Geometry: final body of the model. Coordinates: model frame, mm. Face numbers are marked on the shaded views. A direction names the side the tool comes from. Give positions to 0.01 mm unless a question says otherwise; leave off trailing zeros. Loops run counter-clockwise (first coordinate to the right, second up) from the corner with the lowest first, then second, coordinate; pieces in that order, holes last.
from build123d import *

# Parameters (mm, degrees)
F1_DEPTH = 25.4
F2_R     = 3.425
F3_DEPTH = 25.4
F4_R     = 5.08
F6_DEPTH = 6.35


with BuildPart() as f1:
    # F0 (on Top) → F1 (new body)
    with BuildSketch(Plane.XY):
        with BuildLine():
            ThreePointArc((-17.6783595035, -30.6198168546), (0, -27.3250688074), (17.6783595035, -30.6198168546))
            ThreePointArc((17.6783595035, -30.6198168546), (23.6642037473, -13.6625344037), (35.3567190071, 0))
            ThreePointArc((35.3567190071, 0), (23.6642037473, 13.6625344037), (17.6783595035, 30.6198168546))
            ThreePointArc((17.6783595035, 30.6198168546), (0, 27.3250688074), (-17.6783595035, 30.6198168546))
            ThreePointArc((-17.6783595035, 30.6198168546), (-23.6642037473, 13.6625344037), (-35.3567190071, 0))
            ThreePointArc((-35.3567190071, 0), (-23.6642037473, -13.6625344037), (-17.6783595035, -30.6198168546))
        make_face()
    extrude(amount=F1_DEPTH)

    # F2 (on face) → F3 (cut)
    with BuildSketch(Plane.XY.offset(25.4)):
        Circle(F2_R)
    extrude(amount=-F3_DEPTH, mode=Mode.SUBTRACT)

    # F4
    f4_edges = [f1.edges().sort_by_distance(p)[0] for p in [
        (-35.356719, 0, 12.7),
        (-17.67836, -30.619817, 12.7),
        (17.67836, -30.619817, 12.7),
        (35.356719, 0, 12.7),
        (17.67836, 30.619817, 12.7),
        (-17.67836, 30.619817, 12.7),
        (0, -27.325069, 0),
        (-23.664204, -13.662534, 0),
        (23.664204, -13.662534, 0),
        (-23.664204, 13.662534, 0),
        (23.664204, 13.662534, 0),
        (0, 27.325069, 0),
        (-3.425, 0, 0),
    ]]
    fillet(f4_edges, radius=F4_R)

    # F5 (on face) → F6 (cut)
    with BuildSketch(Plane.XY.offset(25.4)):
        Polygon((-1.9887100499, -6.5160084155), (4.6486737941, -4.9802776317), (6.637383844, 1.5357307838), (1.9887100499, 6.5160084155), (-4.6486737941, 4.9802776317), (-6.637383844, -1.5357307838), align=None)
    extrude(amount=-F6_DEPTH, mode=Mode.SUBTRACT)


solid = f1.part
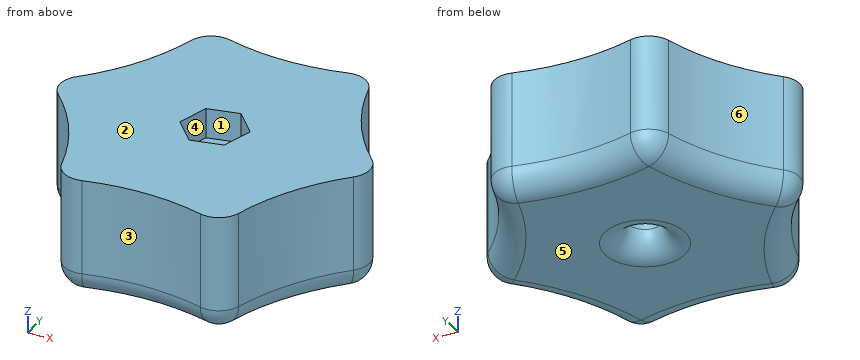
Item 1: Pin query (flat end, axial travel): pin 1 (8 mm diameter, centred on x = 7, z = 18, fed in from -Y); pin 2 (3 mm diameter, centred on x = 4, z = 19, fed in from -Y); pin 3 (1 mm diameter, centred on y = -10, z = 8, fed in from -X). Return the tip coordinate at first contact, or that it passes through.
Values follow:
pin 1: stops at y = -28.57
pin 2: stops at y = -27.63
pin 3: stops at x = -26.36
Item 2: Section query A-A on z = 3. Return loops of the section in (x, y).
Values follow:
outline: (-31.06, -3.27) arc R49.52 cw to (-18.36, -25.27) arc R4.63 ccw to (-12.7, -28.54) arc R49.52 cw to (12.7, -28.54) arc R4.63 ccw to (18.36, -25.27) arc R49.52 cw to (31.06, -3.27) arc R4.63 ccw to (31.06, 3.27) arc R49.52 cw to (18.36, 25.27) arc R4.63 ccw to (12.7, 28.54) arc R49.52 cw to (-12.7, 28.54) arc R4.63 ccw to (-18.36, 25.27) arc R49.52 cw to (-31.06, 3.27) arc R4.63 ccw to start; hole circle Ø7.74 at (0, 0)
Item 3: Section query B-B on x = 0. Return loops of the section in (y, z) (3 decimals).
Values follow:
outline: (-27.325, 5.08) arc R5.08 ccw to (-22.245, 0) - (-8.505, 0) arc R5.08 ccw to (-3.425, 5.08) - (-3.425, 19.05) - (-6.056, 19.05) - (-6.056, 25.4) - (-27.325, 25.4) - close; (3.425, 5.08) arc R5.08 ccw to (8.505, 0) - (22.245, 0) arc R5.08 ccw to (27.325, 5.08) - (27.325, 25.4) - (6.056, 25.4) - (6.056, 19.05) - (3.425, 19.05) - close
Item 4: Draft query along X for the marked faces 3, 4, 5 and 6. Return one class per face: +X half, -X half, draft (parallel to the pull), parting line (faces both ways), or undercut.
Values follow:
face 3: undercut
face 4: undercut
face 5: draft
face 6: -X half
Item 5: Set-up query: the marked faces 1 and 2. Return all of +Z, -Z, +X, -X, +Y, -Y with unobstructed straight access to the full face (end or side cutting, diameter ignored); none if empty.
Values follow:
face 1: +Z
face 2: +Z, +X, -X, +Y, -Y
Item 6: Ray query, probe 1 along X at (y, z) = (13, 10.75); probe 2 along X at (y, z) = (0.5, 19); probe 3 along Y at (x, z) = (1, 14.25). Return the intervals inside material, ascending.
Values follow:
probe 1: x = -24.05 to 24.05
probe 2: x = -32.83 to -3.39, 3.39 to 32.83
probe 3: y = -27.34 to -3.28, 3.28 to 27.34
